Here's how the part is built. I have some questions about the finished solid (model axes, mm). A direction names the side the tool comes from. Round coordinates to 2 decimals unless told otherwise and drop trailing zeros. Write each loop counter-clockwise with the first axis right and the second up, starting at its lowest first coordinate (ties: lowest second). Pieces come first, ordered by that corner, then holes. Notation, with made-up numbers: (-12, -30.5) -> (47, -30.5) arc R28 ccw to (47, 1.5) -> close; hole circle Ø9 at (38, 41.5). An arc over 180 degrees is marked (long way). Answer as CSV lines item,"result".
```python
from build123d import *

# Parameters (mm, degrees)
F1_DEPTH = 175
F3_DEPTH = 25
F4_W     = 110
F4_H     = 50
F5_DEPTH = 22
F6_SIZE  = 3
F7_R     = 7.5
F8_DEPTH = 25


with BuildPart() as f1:
    # F0 (on Front) → F1 (new body, symmetric)
    with BuildSketch(Plane.XZ):
        with BuildLine():
            ThreePointArc((0.0193060127, 12), (3.9707388629, 3.4755758987), (12.7, 0))
            Line((12.7, 0), (36.3, 0))
            ThreePointArc((36.3, 0), (45.0292611371, 3.4755758987), (48.9806939873, 12))
            ThreePointArc((48.9806939873, 12), (45.0292611371, 20.5244241013), (36.3, 24))
            Line((36.3, 24), (12.7, 24))
            ThreePointArc((12.7, 24), (3.9707388629, 20.5244241013), (0.0193060127, 12))
        make_face()
    extrude(amount=F1_DEPTH, both=True)

    # F2 (on face) → F3 (join)
    with BuildSketch(Plane(origin=(0, 0, 0), x_dir=(1, 0, 0), z_dir=(0, 0, -1))):
        Polygon((79.5, 175), (79.5, 200), (79.5, 225), (-30.5, 225), (-30.5, 175), align=None)
    extrude(amount=-F3_DEPTH)

    # F4 (on face) → F5 (cut)
    with BuildSketch(Plane(origin=(0, 0, 0), x_dir=(1, 0, 0), z_dir=(0, 0, -1))):
        with Locations((24.5, 200)):
            Rectangle(F4_W, F4_H)
    extrude(amount=-F5_DEPTH, mode=Mode.SUBTRACT)

    # F6
    f6_edges = [f1.edges().sort_by_distance(p)[0] for p in [
        (24.5, -175, 22),
    ]]
    chamfer(f6_edges, length=F6_SIZE)

    # F7 (on face) → F8 (cut)
    with BuildSketch(Plane(origin=(0, 0, 22), x_dir=(1, 0, 0), z_dir=(0, 0, -1))):
        with Locations((24.5, 200.0529274344)):
            Circle(F7_R)
    extrude(amount=-F8_DEPTH, mode=Mode.SUBTRACT)


solid = f1.part
```
1. Suppose I cut it at B-B on y = 54.5. Please give me the cut outline in (x, z), and give its area (3 significant figures).
Numbers:
outline,"(0.02, 12) arc R12.7 ccw to (12.7, 0) -> (36.3, 0) arc R12.7 ccw to (48.98, 12) arc R12.7 ccw to (36.3, 24) -> (12.7, 24) arc R12.7 ccw to start"
area,"1,040 mm^2"
2. If I drill on line 1 (Y direction, x = 24.5, z = 22.9); line 2 (Z direction, x = 14, y = 157); line 3 (Y direction, x = 24.5, z = 24.25), over which ranges is the centre line in solid material (lowest first)?
Numbers:
line 1,"y = -225 to -207.55, -192.55 to 175"
line 2,"z = 0 to 24"
line 3,"y = -225 to -207.55, -192.55 to -175"
3. On a 3-axis mill with a long thin cutter (end or side, diameter ignored), from which of +Z, -Z, +X, -X, +Y, -Y can I reach the whole of each face in a straight line? I mean faces 1 (the face through (25, -2, 24)), 2 (the face through (24, -211, 25)). Say none if no direction works.
Numbers:
face 1,"+Z, +X, -X, +Y"
face 2,"+Z, +X, -X, +Y, -Y"
4. Suppose I cut it at C-C on x = 73.5. Please give me the cut outline in (y, z), and give its area (3 significant figures).
Numbers:
outline,"(-225, 22) -> (-175, 22) -> (-175, 25) -> (-225, 25) -> close"
area,"150 mm^2"
5. Suppose I cut it at D-D on z = 4.5. Please give me the cut outline in (x, y).
Numbers:
outline,"(3, -175) -> (46, -175) -> (46, 175) -> (3, 175) -> close"
6. Suppose I cut it at A-A on x = 24.5. Please give me the cut outline in (y, z), and give its area (3 significant figures).
Numbers:
outline,"(-225, 22) -> (-207.55, 22) -> (-207.55, 25) -> (-225, 25) -> close; (-192.55, 22) -> (-178, 22) -> (-175, 19) -> (-175, 0) -> (175, 0) -> (175, 24) -> (-175, 24) -> (-175, 25) -> (-192.55, 25) -> close"
area,"8,510 mm^2"
7. For pin 1 Ø12 at (x, y) = (31, 128) entering from +Z; pin 2 Ø5 at (y, z) = (-126.5, 22.5) entering from -X; pin 3 Ø1 at (y, z) = (16, 7) entering from +X, each with a flat end and sliding along its axis, tell me the tip position at first contact or that it passes through.
Numbers:
pin 1,"stops at z = 24"
pin 2,"stops at x = 3.45"
pin 3,"stops at x = 47.89"
8. If we mould it in two halves opening along Y, with no side actions, what happens to faces 3 (the face through (22.874, -192.731, 23.479)), 4 (the face through (3.87, -2.45, 3.57)), 5 (the face through (24, -175, 9))? For each: released by +Y, released by -Y, zero draft, split by the parting line, or undercut.
Numbers:
face 3,"undercut"
face 4,"zero draft"
face 5,"released by -Y"
